from build123d import *

# Parameters (mm, degrees)
BOSS_EXTRU_1_DEPTH      = 18
BOSS_EXTRU_1_DEPTH_BACK = 18


with BuildPart() as part:
    # Esquisse1 → Boss.-Extru.1 (new body, two sides)
    with BuildSketch(Plane.XY) as boss_extru_1_sk:
        Polygon((0, 0), (0, 80), (25.711504387, 110.641777725), (28.009637717, 108.713414896), (3.916221868, 80), (3.916221868, 0), align=None)
    extrude(amount=BOSS_EXTRU_1_DEPTH)
    extrude(boss_extru_1_sk.sketch, amount=-BOSS_EXTRU_1_DEPTH_BACK)


solid = part.part
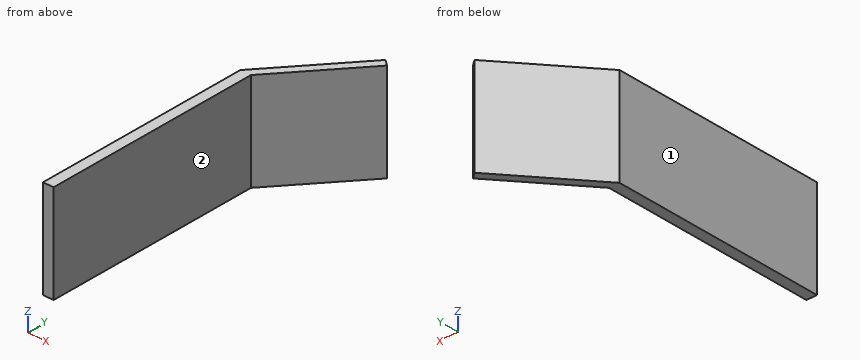
Design review of the part built by this model. Coordinates are the model's own, in mm. Face numbers are marked on the shaded views. A direction names the side the tool comes from. Give positions to 0.01 mm unless a question says otherwise; leave off trailing zeros. Write each loop counter-clockwise with the first axis right and the second up, starting at its lowest first coordinate (ties: lowest second). Pieces come first, ordered by that corner, then holes. Notation, with made-up numbers: M -15,-32.5 L -8,-32.5 A26 ccw -8,-10.5 Z; hole C -8.75,38.5 d5. An arc over 180 degrees is marked long. Return JSON: item names as keys, results as strings. Group by question number.
Item 1: Clearance check with flat-ended pins moving along their axes: pin 1 Ø8 at (x, z) = (17, 8) entering from +Y; pin 2 Ø6 at (x, z) = (19, -1) entering from -Y; pin 3 Ø4 at (x, z) = (23, 2.5) entering from -Y. State where each tip first meets the part, or that it passes through.
Item 2: Take a section at A-A (y = 42). Give the boundary of the cut face in (x, z).
Item 3: Tool access review of the marked faces 1 and 2: name each direction out of +Z, -Z, +X, -X, +Y, -Y from which nothing blocks a thin tool from reaching the whole face with its end or side.
Item 4: Take a section at B-B (z = 4). Give the boundary of the cut face in (x, y), plus the area to 3 significant figures.
Item 5: Wall thickness on line 1 along X through (y, z) = (29, -9); line 2 along Y through (x, z) = (20.25, 14); line 3 along Y through (x, z) = (11, 5): over which ranges is each line inside the solid? List them lowest first.
Item 6: Take a section at C-C (x = 2.5). Give the boundary of the cut face in (y, z), plus the area to 3 significant figures.
Return value:
{
 "1": {"pin 1": "stops at y = 105.03", "pin 2": "stops at y = 94.4", "pin 3": "stops at y = 100.36"},
 "2": {"outline": "M 0,-18 L 3.92,-18 L 3.92,18 L 0,18 Z"},
 "3": {"face 1": "+Z, -Z, -X, +Y, -Y", "face 2": "+Z, -Z, +X, -Y"},
 "4": {"outline": "M 0,0 L 3.92,0 L 3.92,80 L 28.01,108.71 L 25.71,110.64 L 0,80 Z", "area": "430 mm2"},
 "5": {"line 1": "x = 0 to 3.92", "line 2": "y = 99.47 to 104.13", "line 3": "y = 88.44 to 93.11"},
 "6": {"outline": "M 0,-18 L 82.98,-18 L 82.98,18 L 0,18 Z", "area": "2,990 mm2"}
}
